Can you work these out from the model? Positions are in its coordinate system, mm. Face numbers are marked on the shaded views. Give positions to 0.01 mm unless a question says otherwise; leave off trailing zeros. Write each loop counter-clockwise with the first axis right and the second up, starting at its lowest first coordinate (ties: lowest second). Pieces come first, ordered by that corner, then holes. Notation, with made-up numbers: M -1.5,34.25 L 27.5,34.25 A20 cw 27.5,38.25 Z; hole C 88,62 d9. An arc over 180 degrees is marked long. Write each question's results on one line, items separated by ' | '.
from build123d import *

# Parameters (mm, degrees)
SKETCH1_W           = 266
SKETCH1_H           = 213.3
BOSS_EXTRUDE1_DEPTH = 7.5
SKETCH2_W           = 242
SKETCH2_H           = 189
CUT_EXTRUDE1_DEPTH  = 5
CUT_EXTRUDE2_DEPTH  = 5
FILLET1_R           = 5
FILLET2_R           = 10


with BuildPart() as part:
    # Sketch1 → Boss-Extrude1 (new body)
    with BuildSketch(Plane(origin=(0, 0, 0), x_dir=(1, 0, 0), z_dir=(0, 1, 0))):
        with Locations((133, 106.65)):
            Rectangle(SKETCH1_W, SKETCH1_H)
    extrude(amount=BOSS_EXTRUDE1_DEPTH)

    # Sketch2 → Cut-Extrude1 (cut)
    with BuildSketch(Plane(origin=(0, 7.5, 0), x_dir=(1, 0, 0), z_dir=(0, 1, 0))):
        with Locations((133, 106.65)):
            Rectangle(SKETCH2_W, SKETCH2_H)
    extrude(amount=-CUT_EXTRUDE1_DEPTH, mode=Mode.SUBTRACT)

    # Sketch3 → Cut-Extrude2 (cut)
    with BuildSketch(Plane(origin=(0, 7.5, 0), x_dir=(1, 0, 0), z_dir=(0, 1, 0))):
        Polygon((12, 194.078932188), (4.5, 201.578932188), (4.5, 208.8), (11.421067812, 208.8), (19.071067812, 201.15), align=None)
        Polygon((19.071067812, 12.15), (12, 19.221067812), (4.5, 11.721067812), (4.5, 4.5), (11.421067812, 4.5), align=None)
        Polygon((254, 19.221067812), (261.5, 11.721067812), (261.5, 4.5), (254.578932188, 4.5), (246.928932188, 12.15), align=None)
        Polygon((246.928932188, 201.15), (254, 194.078932188), (261.5, 201.578932188), (261.5, 208.8), (254.578932188, 208.8), align=None)
    extrude(amount=-CUT_EXTRUDE2_DEPTH, mode=Mode.SUBTRACT)

    # Fillet1
    fillet1_edges = [part.edges().sort_by_distance(p)[0] for p in [
        (4.5, 5, -208.8),
        (4.5, 5, -4.5),
        (261.5, 5, -4.5),
        (261.5, 5, -208.8),
    ]]
    fillet(fillet1_edges, radius=FILLET1_R)

    # Fillet2
    fillet2_edges = [part.edges().sort_by_distance(p)[0] for p in [
        (0, 3.75, -213.3),
        (266, 3.75, -213.3),
        (266, 3.75, 0),
        (0, 3.75, 0),
    ]]
    fillet(fillet2_edges, radius=FILLET2_R)


solid = part.part
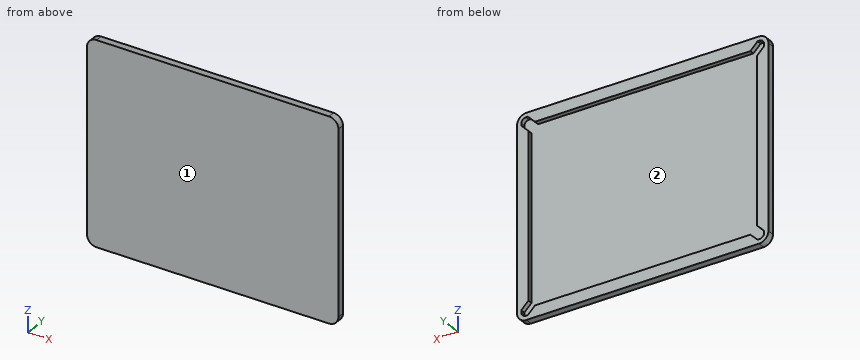
Item 1: Thinking about a two-plate mould opening in Z: for the marked faces 1 and 2, which applies, +Z half, -Z half, draft (parallel to the pull), parting line (faces both ways), or undercut?
Geometry says:
face 1: draft | face 2: undercut
Item 2: I want a section at C-C, the plane z = -111. Please give me the cut outline in (x, y), and give its area (3 significant figures).
Geometry says:
outline: M 0,0 L 266,0 L 266,7.5 L 254,7.5 L 254,2.5 L 12,2.5 L 12,7.5 L 0,7.5 Z | area: 785 mm2
Item 3: I'm going to push a flat-ended pin straight in: pin 1 (10 mm diameter, centred on x = 81, z = -142.5, fed in from +Y). Where does the tip first touch, or does it pass through?
Geometry says:
pin 1: stops at y = 2.5
Item 4: I want a section at B-B, the plane x = 200. Please give me the cut outline in (y, z), and give its area (3 significant figures).
Geometry says:
outline: M 0,-213.3 L 7.5,-213.3 L 7.5,-201.15 L 2.5,-201.15 L 2.5,-12.15 L 7.5,-12.15 L 7.5,0 L 0,0 Z | area: 655 mm2
Item 5: If I drill on line 1 (Z direction, x = 238.5, y = 4.5); line 2 (X direction, y = 3.5, z = -49); line 3 (X direction, y = 6, z = -10.5), over which ranges is the centre line in solid material (lowest first)? Write a range as from..to.
Geometry says:
line 1: z = -213.3..-201.15, -12.15..0 | line 2: x = 0..12, 254..266 | line 3: x = 0..4.5, 17.42..248.58, 261.5..266
